from build123d import *

# Parameters (mm, degrees)
SKETCH1_R           = 3.3
BOSS_EXTRUDE1_DEPTH = 4.7625
FILLET1_R           = 0.254


with BuildPart() as part:
    # Sketch1 → Boss-Extrude1 (new body)
    with BuildSketch(Plane(origin=(0, 0, 0), x_dir=(1, 0, 0), z_dir=(0, 1, 0))):
        with BuildLine():
            Line((16.658671, -23.484448), (-6.055469, -11.163391))
            ThreePointArc((-6.055469, -11.163391), (10.341596, -7.371661), (8.57781, 9.365425))
            Line((8.57781, 9.365425), (27.63363, -8.087836))
            ThreePointArc((27.63363, -8.087836), (28.95647, -20.64065), (16.658671, -23.484448))
        make_face()
        with Locations((21.200273, -15.111905)):
            Circle(SKETCH1_R, mode=Mode.SUBTRACT)
    extrude(amount=BOSS_EXTRUDE1_DEPTH)

    # Fillet1
    fillet1_edges = [part.edges().sort_by_distance(p)[0] for p in [
        (-6.055469, 2.38125, 11.163391),
        (8.57781, 2.38125, -9.365425),
    ]]
    fillet(fillet1_edges, radius=FILLET1_R)


solid = part.part
Can you work these out from the model? Positions are in its coordinate system, mm. Give positions to 0.01 mm unless a question says otherwise; leave off trailing zeros. Loops run counter-clockwise (first coordinate to the right, second up) from the corner with the lowest first, then second, coordinate; pieces in that order, holes last. Notation, with made-up numbers: (14, 61.25) -> (47, 61.25) arc R24 cw to (47, 93.25) -> close; hole circle Ø9 at (54.5, 46). An arc over 180 degrees is marked (long way). Return JSON: item names as keys, results as strings.
Q1. I want a section at C-C, the plane y = 4.1. List the corners of the cut face in (x, z) for me (3 decimals).
Checks:
{"outline": "(-2.898, 12.876) arc R0.254 ccw to (-2.722, 12.405) arc R12.7 cw to (10.838, -6.62) arc R0.254 ccw to (11.227, -6.939) -> (27.634, 8.088) arc R9.525 ccw to (16.659, 23.484) -> close; hole circle Ø6.6 at (21.2, 15.112)"}
Q2. We'd pull the mould along Z, two halves only. Please class faces 1 (the face through (17.903, 2.348, 14.967)), 2 (the face through (18, 4.762, 12)), 3 (the face through (29.07, 2.35, 20.48)), 4 (the face through (10.22, 2.35, 7.54)): released by +Z, released by -Z, zero draft, split by the parting line, or undercut.
Checks:
{"face 1": "undercut", "face 2": "zero draft", "face 3": "split by the parting line", "face 4": "undercut"}
Q3. I want a section at D-D, the plane z = 22. List the corners of the cut face in (x, y) for me, then the cut area to 3 significant figures.
Checks:
{"outline": "(13.92, 0) -> (27.78, 0) -> (27.78, 4.76) -> (13.92, 4.76) -> close", "area": "66.0 mm2"}
Q4. For pin 1 Ø1.5 at (x, y) = (10, 1.5) entering from -Z, with a flat end and sliding along its axis, tell me the tip position at first contact or that it passes through.
Checks:
{"pin 1": "stops at z = 6.76"}
Q5. I want a section at B-B, the plane z = 16.5. List the corners of the cut face in (x, y) for me.
Checks:
{"outline": "(3.78, 0) -> (18.21, 0) -> (18.21, 4.76) -> (3.78, 4.76) -> close; (24.19, 0) -> (30.62, 0) -> (30.62, 4.76) -> (24.19, 4.76) -> close"}
Q6. I want a section at A-A, the plane x = 23. List the corners of the cut face in (y, z) for me.
Checks:
{"outline": "(0, 3.84) -> (4.76, 3.84) -> (4.76, 12.35) -> (0, 12.35) -> close; (0, 17.88) -> (4.76, 17.88) -> (4.76, 24.47) -> (0, 24.47) -> close"}
Q7. I need wall thicknesses on probe 1 along X at (y, z) = (1.35, 17); probe 2 along X at (y, z) = (2.45, 13); probe 3 along X at (y, z) = (4.35, -3.5). Which ranges of each line are inside material? Lowest first, please.
Checks:
{"probe 1": "x = 4.7 to 18.49, 23.91 to 30.54", "probe 2": "x = -2.67 to 18.66, 23.74 to 30.49", "probe 3": "x = 12.21 to 14.98"}
